from build123d import *

# Parameters (mm, degrees)
F1_DEPTH = 15


with BuildPart() as f1:
    # F0 (on Front) → F1 (new body)
    with BuildSketch(Plane.XZ):
        with BuildLine():
            Line((-20, 30), (-30, 30))
            Line((-30, 30), (-44.90712, 13.333333))
            ThreePointArc((-44.90712, 13.333333), (-50, 0), (-44.90712, -13.333333))
            Line((-44.90712, -13.333333), (-30, -30))
            Line((-30, -30), (-17.320508, -30))
            ThreePointArc((-17.320508, -30), (0, -20), (17.320508, -30))
            Line((17.320508, -30), (30, -30))
            Line((30, -30), (30, 30))
            Line((30, 30), (20, 30))
            Line((20, 30), (0, 0))
            Line((0, 0), (-20, 30))
        make_face()
    extrude(amount=F1_DEPTH)


solid = f1.part
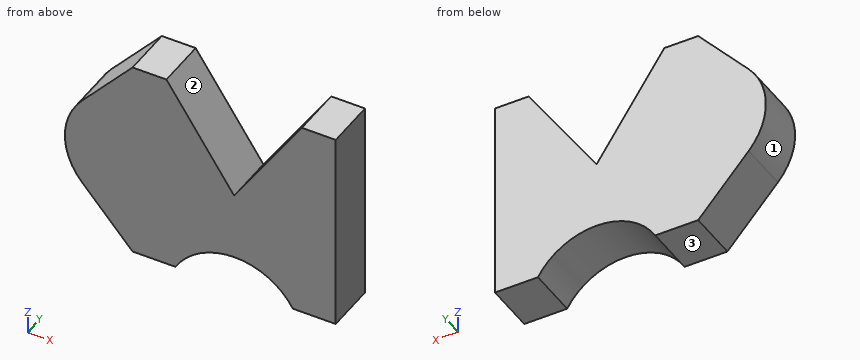
Source: CAD feature listing. Evaluate the final solid. Frame: model axes, mm. Face numbers are marked on the shaded views. Give positions to 0.01 mm unless a question says otherwise; leave off trailing zeros. Order: outer loops, then holes, each group sorted by start corner. A loop starts at its lowest first (then second) coordinate and runs counter-clockwise, first axis right, second up. Notation, with made-up numbers: (3, 28.5) -> (41, 28.5) arc R19 ccw to (41, 39.5) -> close; hole circle Ø3 at (37.5, -11). An arc over 180 degrees is marked (long way). Write item = value, one per line.
Item 1: Section query B-B (z = -24). Output: boundary loops of the cut face in (x, y).
Check result:
outline = (-35.37, -15) -> (-12, -15) -> (-12, 0) -> (-35.37, 0) -> close; (12, -15) -> (30, -15) -> (30, 0) -> (12, 0) -> close
Item 2: Contact query for flat-ended pins moving along their axis: pin 1 (5 mm diameter, centred on x = 4.5, y = -7.5, fed in from -Z) (3 decimals); pin 2 (6 mm diameter, centred on y = -7, z = -8.5, fed in from -X); pin 3 (6 mm diameter, centred on y = -11, z = 19, fed in from -X). Output: stop coordinate, or through.
Check result:
pin_1 = -21.265
pin_2 = -49.23
pin_3 = -42.52
Item 3: Section query C-C (z = 16.5). Output: boundary loops of the cut face in (x, y), then the cut area to 3 significant figures.
Check result:
outline = (-42.07, -15) -> (-11, -15) -> (-11, 0) -> (-42.07, 0) -> close; (11, -15) -> (30, -15) -> (30, 0) -> (11, 0) -> close
area = 751 mm²
Item 4: Section query D-D (x = -12). Output: boundary loops of the cut face in (y, z), then the cut area to 3 significant figures.
Check result:
outline = (-15, -24) -> (0, -24) -> (0, 18) -> (-15, 18) -> close
area = 630 mm²
Item 5: Section query A-A (y = -11.25). Output: boundary loops of the cut face in (x, z).
Check result:
outline = (-44.91, -13.33) -> (-30, -30) -> (-17.32, -30) arc R20 cw to (17.32, -30) -> (30, -30) -> (30, 30) -> (20, 30) -> (0, 0) -> (-20, 30) -> (-30, 30) -> (-44.91, 13.33) arc R20 ccw to start
Item 6: Mould query, pull axis X, two halves, no side actions, for the marked faces 1, 2 and 3. Classes: +X half, -X half, draft (parallel to the pull), parting line (faces both ways), or undercut.
Check result:
face_1 = -X half
face_2 = undercut
face_3 = draft
Item 7: Ray query, probe 1 along X at (y, z) = (-9.5, 27); probe 2 along X at (y, z) = (-10.5, 5); probe 3 along X at (y, z) = (-2.25, -9). Return the intervals inside material, ascending.
Check result:
probe_1 = -32.68 to -18, 18 to 30
probe_2 = -49.36 to -3.33, 3.33 to 30
probe_3 = -47.86 to 30
